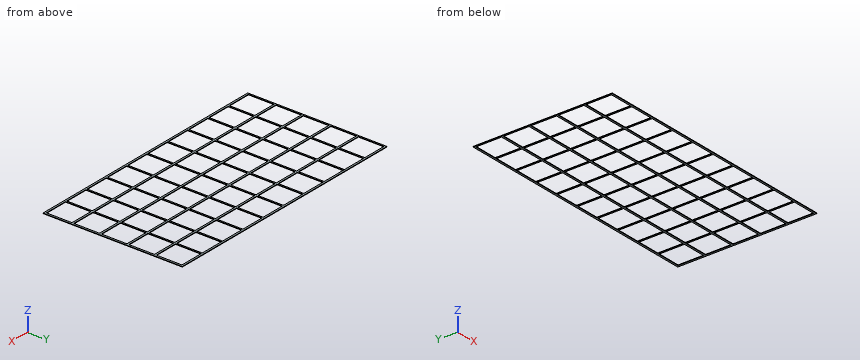
```python
from build123d import *

# Parameters (mm, degrees)
SKETCH1_W           = 1695.45
SKETCH1_H           = 933.45
BOSS_EXTRUDE1_DEPTH = 3.175
SKETCH2_W           = 158.75
SKETCH2_H           = 171.45
CUT_EXTRUDE1_DEPTH  = 4.175


with BuildPart() as part:
    # Sketch1 → Boss-Extrude1 (new body)
    with BuildSketch(Plane.XY):
        Rectangle(SKETCH1_W, SKETCH1_H)
    extrude(amount=BOSS_EXTRUDE1_DEPTH)

    # Sketch2 → Cut-Extrude1 (cut, through all)
    with BuildSketch(Plane.XY.offset(3.175)):
        with Locations((-758.825, 368.3)):
            Rectangle(SKETCH2_W, SKETCH2_H)
        with Locations((-590.55, 368.3)):
            Rectangle(SKETCH2_W, SKETCH2_H)
        with Locations((-422.275, 368.3)):
            Rectangle(SKETCH2_W, SKETCH2_H)
        with Locations((-254, 368.3)):
            Rectangle(SKETCH2_W, SKETCH2_H)
        with Locations((-85.725, 368.3)):
            Rectangle(SKETCH2_W, SKETCH2_H)
        with Locations((82.55, 368.3)):
            Rectangle(SKETCH2_W, SKETCH2_H)
        with Locations((250.825, 368.3)):
            Rectangle(SKETCH2_W, SKETCH2_H)
        with Locations((419.1, 368.3)):
            Rectangle(SKETCH2_W, SKETCH2_H)
        with Locations((587.375, 368.3)):
            Rectangle(SKETCH2_W, SKETCH2_H)
        with Locations((755.65, 368.3)):
            Rectangle(SKETCH2_W, SKETCH2_H)
        with Locations((-590.55, 184.15)):
            Rectangle(SKETCH2_W, SKETCH2_H)
        with Locations((-422.275, 184.15)):
            Rectangle(SKETCH2_W, SKETCH2_H)
        with Locations((-254, 184.15)):
            Rectangle(SKETCH2_W, SKETCH2_H)
        with Locations((-85.725, 184.15)):
            Rectangle(SKETCH2_W, SKETCH2_H)
        with Locations((82.55, 184.15)):
            Rectangle(SKETCH2_W, SKETCH2_H)
        with Locations((250.825, 184.15)):
            Rectangle(SKETCH2_W, SKETCH2_H)
        with Locations((419.1, 184.15)):
            Rectangle(SKETCH2_W, SKETCH2_H)
        with Locations((587.375, 184.15)):
            Rectangle(SKETCH2_W, SKETCH2_H)
        with Locations((755.65, 184.15)):
            Rectangle(SKETCH2_W, SKETCH2_H)
        with Locations((-590.55, 0)):
            Rectangle(SKETCH2_W, SKETCH2_H)
        with Locations((-422.275, 0)):
            Rectangle(SKETCH2_W, SKETCH2_H)
        with Locations((-254, 0)):
            Rectangle(SKETCH2_W, SKETCH2_H)
        with Locations((-85.725, 0)):
            Rectangle(SKETCH2_W, SKETCH2_H)
        with Locations((82.55, 0)):
            Rectangle(SKETCH2_W, SKETCH2_H)
        with Locations((250.825, 0)):
            Rectangle(SKETCH2_W, SKETCH2_H)
        with Locations((419.1, 0)):
            Rectangle(SKETCH2_W, SKETCH2_H)
        with Locations((587.375, 0)):
            Rectangle(SKETCH2_W, SKETCH2_H)
        with Locations((755.65, 0)):
            Rectangle(SKETCH2_W, SKETCH2_H)
        with Locations((-590.55, -184.15)):
            Rectangle(SKETCH2_W, SKETCH2_H)
        with Locations((-422.275, -184.15)):
            Rectangle(SKETCH2_W, SKETCH2_H)
        with Locations((-254, -184.15)):
            Rectangle(SKETCH2_W, SKETCH2_H)
        with Locations((-85.725, -184.15)):
            Rectangle(SKETCH2_W, SKETCH2_H)
        with Locations((82.55, -184.15)):
            Rectangle(SKETCH2_W, SKETCH2_H)
        with Locations((250.825, -184.15)):
            Rectangle(SKETCH2_W, SKETCH2_H)
        with Locations((419.1, -184.15)):
            Rectangle(SKETCH2_W, SKETCH2_H)
        with Locations((587.375, -184.15)):
            Rectangle(SKETCH2_W, SKETCH2_H)
        with Locations((755.65, -184.15)):
            Rectangle(SKETCH2_W, SKETCH2_H)
        with Locations((-590.55, -368.3)):
            Rectangle(SKETCH2_W, SKETCH2_H)
        with Locations((-422.275, -368.3)):
            Rectangle(SKETCH2_W, SKETCH2_H)
        with Locations((-254, -368.3)):
            Rectangle(SKETCH2_W, SKETCH2_H)
        with Locations((-85.725, -368.3)):
            Rectangle(SKETCH2_W, SKETCH2_H)
        with Locations((82.55, -368.3)):
            Rectangle(SKETCH2_W, SKETCH2_H)
        with Locations((250.825, -368.3)):
            Rectangle(SKETCH2_W, SKETCH2_H)
        with Locations((419.1, -368.3)):
            Rectangle(SKETCH2_W, SKETCH2_H)
        with Locations((587.375, -368.3)):
            Rectangle(SKETCH2_W, SKETCH2_H)
        with Locations((755.65, -368.3)):
            Rectangle(SKETCH2_W, SKETCH2_H)
        with Locations((-758.825, 184.15)):
            Rectangle(SKETCH2_W, SKETCH2_H)
        with Locations((-758.825, 0)):
            Rectangle(SKETCH2_W, SKETCH2_H)
        with Locations((-758.825, -184.15)):
            Rectangle(SKETCH2_W, SKETCH2_H)
        with Locations((-758.825, -368.3)):
            Rectangle(SKETCH2_W, SKETCH2_H)
    extrude(amount=-CUT_EXTRUDE1_DEPTH, mode=Mode.SUBTRACT)


solid = part.part
```
Design review of the part built by this model. Coordinates are the model's own, in mm. Round coordinates to 2 decimals unless told otherwise and drop trailing zeros. Write each loop counter-clockwise with the first axis right and the second up, starting at its lowest first coordinate (ties: lowest second). Pieces come first, ordered by that corner, then holes. Notation, with made-up numbers: (-20.75, -32.5) -> (-12.75, -32.5) arc R16 ccw to (-12.75, -24.5) -> close; hole circle Ø4 at (73.5, 78). An arc over 180 degrees is marked (long way). Answer in a Markdown table with one row per item.
Q1. To check wall thickness, follow L1, parallel to Y at x = 682, z = 2.6 (3 decimals). State the ranges of the line that lie inside material, in increasing order. Write a range as [from, to].
The answers:
| item | result |
|---|---|
| L1 | [-466.725, -454.025], [-282.575, -269.875], [-98.425, -85.725], [85.725, 98.425], [269.875, 282.575], [454.025, 466.725] |
Q2. Take a section at B-B, the plane y = 410.5. Count the separate pieces of the cut face and the enclosed holes in it, then the cut area to 3 significant figures.
The answers:
| item | result |
|---|---|
| separate pieces | 11 |
| enclosed holes | 0 |
| area | 343 mm² |
Q3. Take a section at A-A, the plane x = 583.5. State the section outline as (y, z) points (3 decimals), then the cut area to 3 significant figures.
The answers:
| item | result |
|---|---|
| outline | (-466.725, 0) -> (-454.025, 0) -> (-454.025, 3.175) -> (-466.725, 3.175) -> close; (-282.575, 0) -> (-269.875, 0) -> (-269.875, 3.175) -> (-282.575, 3.175) -> close; (-98.425, 0) -> (-85.725, 0) -> (-85.725, 3.175) -> (-98.425, 3.175) -> close; (85.725, 0) -> (98.425, 0) -> (98.425, 3.175) -> (85.725, 3.175) -> close; (269.875, 0) -> (282.575, 0) -> (282.575, 3.175) -> (269.875, 3.175) -> close; (454.025, 0) -> (466.725, 0) -> (466.725, 3.175) -> (454.025, 3.175) -> close |
| area | 242 mm² |
